Source: CAD feature listing. Evaluate the final solid. Frame: model axes, mm. A direction names the side the tool comes from. Coordinates: 2 decimals unless noted, no trailing zeros. Order: outer loops, then holes, each group sorted by start corner. A loop starts at its lowest first (then second) coordinate and runs counter-clockwise, first axis right, second up.
```python
from build123d import *

# Parameters (mm, degrees)
F1_DEPTH = 4
F2_W     = 6
F2_H     = 3
F3_DEPTH = 3
F6_DEPTH = 4.0099186287


with BuildPart() as f1:
    # F0 (on Front) → F1 (new body)
    with BuildSketch(Plane.XZ):
        with BuildLine():
            Line((0, 5), (0, 0))
            Line((0, 0), (6, 0))
            Line((6, 0), (6, 5))
            Line((6, 5), (5, 5))
            ThreePointArc((5, 5), (3.5, 3.5), (2, 5))
            Line((2, 5), (0, 5))
        make_face()
    extrude(amount=F1_DEPTH)

    # F2 (on face) → F3 (cut)
    with BuildSketch(Plane.XZ.offset(4)):
        with Locations((3, 3.5)):
            Rectangle(F2_W, F2_H)
    extrude(amount=-F3_DEPTH, mode=Mode.SUBTRACT)

    # F5 (on 3pt) → F6 (cut, through all)
    with BuildSketch(Plane(origin=(1, -2, 3), x_dir=(0.9636241117, 0.1482498633, -0.222374795), z_dir=(-0.2672612419, 0.5345224838, -0.8017837257))):
        Polygon((5.1887452166, 3.3282011774), (-1.0377490433, 2.2188007849), (5.1887452166, -0.2773500981), align=None)
    extrude(amount=-F6_DEPTH, mode=Mode.SUBTRACT)


solid = f1.part
```
Q1. Section query C-C on z = 0.6. Output: boundary loops of the cut face in (x, y).
Solutions:
outline: (0, -4) - (4.2, -4) - (6, -3.1) - (6, 0) - (0, 0) - close
Q2. Pin query (flat end, axial travel): P1, Ø3, axis at x = 4.5, z = 3, coming from the +Y side; P2, Ø1.5, axis at x = 3.5, y = -2.5, coming from the +Z side; P3, Ø0.9, axis at x = 4, z = 3, coming from the -Y side. Return the tip coordinate at first contact, or that it passes through.
Solutions:
P1: stops at y = 0
P2: stops at z = 2
P3: stops at y = -1
Q3. Section query B-B on x = 1.5. Output: boundary loops of the cut face in (y, z), plus the area to 3 significant figures.
Solutions:
outline: (-4, 0) - (0, 0) - (0, 5) - (-1, 5) - (-1, 2) - (-3.25, 2) - (-4, 1.5) - close
area: 10.8 mm2
Q4. Section query A-A on z = 4.1. Output: boundary loops of the cut face in (x, y), plus the area to 3 significant figures.
Solutions:
outline: (0, -1) - (2.3, -1) - (2.3, 0) - (0, 0) - close; (4.7, -1) - (6, -1) - (6, 0) - (4.7, 0) - close
area: 3.60 mm2
Q5. Section query D-D on y = -3.65. Output: boundary loops of the cut face in (x, z), plus the area to 3 significant figures.
Solutions:
outline: (0, 0) - (6, 0) - (6, 0.23) - (0.7, 2) - (0, 2) - close
area: 7.32 mm2
Q6. Material intervals for line 1 along Y through (x, z) = (4.25, 3.05); line 2 along Z through (x, y) = (3.5, -1.6); line 3 along X through (y, z) = (-0.5, 4.7), sorted ascending.
Solutions:
line 1: y = -1 to 0
line 2: z = 0 to 2
line 3: x = 0 to 2.03, 4.97 to 6
Q7. Pull-direction query (X, two-part tool) for faces 1 (the flat face through (2, -4, 1)), 2 (the cylindrical face through (3.5, -0.5, 3.5)), 3 (the flat face through (3.625, -2.886, 1.534)); classes: pulls with the +X half, pulls with the -X half, needs draft (parallel to the pull), parting line crosses it, or undercut.
Solutions:
face 1: needs draft
face 2: undercut
face 3: pulls with the +X half
Q8. Set-up query: faces 4 (the flat face through (0, -2, 1)), 5 (the flat face through (3, -1, 3)). Return all of +Z, -Z, +X, -X, +Y, -Y with unobstructed straight access to the full face (end or side cutting, diameter ignored); none if empty.
Solutions:
face 4: +Z, -Z, -X, +Y, -Y
face 5: +Z, +X, -X, -Y
